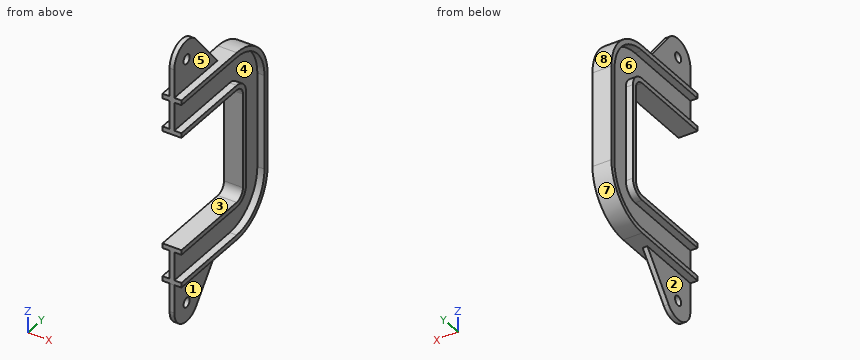
from build123d import *

# Parameters (mm, degrees)
F3_R     = 5
F4_DEPTH = 2.5


with BuildPart() as f2:
    # F2: sweep along a path in F1
    with BuildLine(Plane.YZ) as f2_path:
        Line((0, -20), (90, -20))
        ThreePointArc((90, -20), (97.071068, -22.928932), (100, -30))
        Line((100, -30), (100, -130))
        ThreePointArc((100, -130), (97.071068, -137.071068), (90, -140))
        Line((90, -140), (0, -140))
    # F0 (on Front) → F2 (sweep)
    with BuildSketch(Plane.XZ):
        Polygon((2.5, -12), (2.5, 0), (2.5, 12), (2.5, 15), (5.5, 15), (10, 15), (10, 20), (0, 20), (-10, 20), (-10, 15), (-5.5, 15), (-2.5, 15), (-2.5, 12), (-2.5, 0), (-2.5, -12), (-2.5, -15), (-5.5, -15), (-10, -15), (-10, -20), (0, -20), (10, -20), (10, -15), (5.5, -15), (2.5, -15), align=None)
    sweep(path=f2_path.line)

    # F3 (on Right) → F4 (join, symmetric)
    with BuildSketch(Plane.YZ):
        with BuildLine():
            Line((0, 50), (0, 20))
            Line((0, 20), (70, 20))
            Line((70, 20), (35.548045, 62.580075))
            ThreePointArc((35.548045, 62.580075), (13.327703, 68.854189), (0, 50))
        make_face()
        with Locations((20, 50)):
            Circle(F3_R, mode=Mode.SUBTRACT)
        with BuildLine():
            Line((0, -180), (0, -210))
            ThreePointArc((0, -210), (13.327703, -228.854189), (35.548045, -222.580075))
            Line((35.548045, -222.580075), (70, -180))
            Line((70, -180), (0, -180))
        make_face()
        with Locations((20, -210)):
            Circle(F3_R, mode=Mode.SUBTRACT)
    extrude(amount=F4_DEPTH, both=True)


solid = f2.part
Here's how the part is built. I have some questions about the finished solid (model axes, mm). Face numbers are marked on the shaded views. A direction names the side the tool comes from. Coordinates: 2 decimals unless noted, no trailing zeros. Write each loop counter-clockwise with the first axis right and the second up, starting at its lowest first coordinate (ties: lowest second). Pieces come first, ordered by that corner, then holes.
1) If we section it at A-A (x = -5.5): List the corners of the cut face in (y, z) for me.
Filled in:
outline: (0, -180) - (90, -180) arc R50 ccw to (140, -130) - (140, -30) arc R50 ccw to (90, 20) - (0, 20) - (0, 15) - (90, 15) arc R45 cw to (135, -30) - (135, -130) arc R45 cw to (90, -175) - (0, -175) - close; (0, -145) - (90, -145) arc R15 ccw to (105, -130) - (105, -30) arc R15 ccw to (90, -15) - (0, -15) - (0, -20) - (90, -20) arc R10 cw to (100, -30) - (100, -130) arc R10 cw to (90, -140) - (0, -140) - close
2) If I drill on line 1 (Z direction, x = -3.25, y = 14.5); line 2 (Z direction, x = 0.35, y = 20); line 3 (Y direction, x = 8.25, z = -50.5), over which ranges is the centre line in solid material (lowest first)?
Filled in:
line 1: z = -180 to -175, -145 to -140, -20 to -15, 15 to 20
line 2: z = -230 to -215, -205 to -140, -20 to 45, 55 to 70
line 3: y = 100 to 105, 135 to 140
3) Which directions (+Z, -Z, +X, -X, +Y, -Y) give clear straight access to the entire face, cutting with the end or side of a thin tool? Please do the marked faces 1, 2, 3 and 4.
Filled in:
face 1: -Z, +X, +Y, -Y
face 2: -Z, -X, +Y, -Y
face 3: +X, -X, -Y
face 4: +X
4) I'm going to push flat-ended pins straight in: pin 1 (4 mm diameter, centred on x = 4, z = -158, fed in from +Y); pin 2 (6 mm diameter, centred on x = -1.5, y = 48, fed in from -Z); pin 3 (8 mm diameter, centred on y = 22, z = -188, fed in from -X). Where does each tip first touch, or does it pass through?
Filled in:
pin 1: stops at y = 132.71
pin 2: stops at z = -210.9
pin 3: stops at x = -2.5
5) Thinking about a two-plate mould opening in Z: for the marked faces 5, 6, 7 and 8, which applies, +Z half, -Z half, draft (parallel to the pull), parting line (faces both ways), or undercut?
Filled in:
face 5: draft
face 6: undercut
face 7: -Z half
face 8: +Z half
6) If we section it at C-C (z = -151.5): List the corners of the cut face in (x, y) for me.
Filled in:
outline: (-10, 129.53) - (-2.5, 129.53) - (-2.5, 0) - (2.5, 0) - (2.5, 129.53) - (10, 129.53) - (10, 135.14) - (-10, 135.14) - close
